Source: three-view drawing plus pictorial views. Frame: mm from the lowest corner of the part. Give positions to 0.01 mm unless a question says otherwise; leave off trailing zeros. Write each loop counter-clockwise with the first axis right and the second up, starting at its lowest first coordinate (ties: lowest second). Pieces come first, ordered by that corner, then holes.
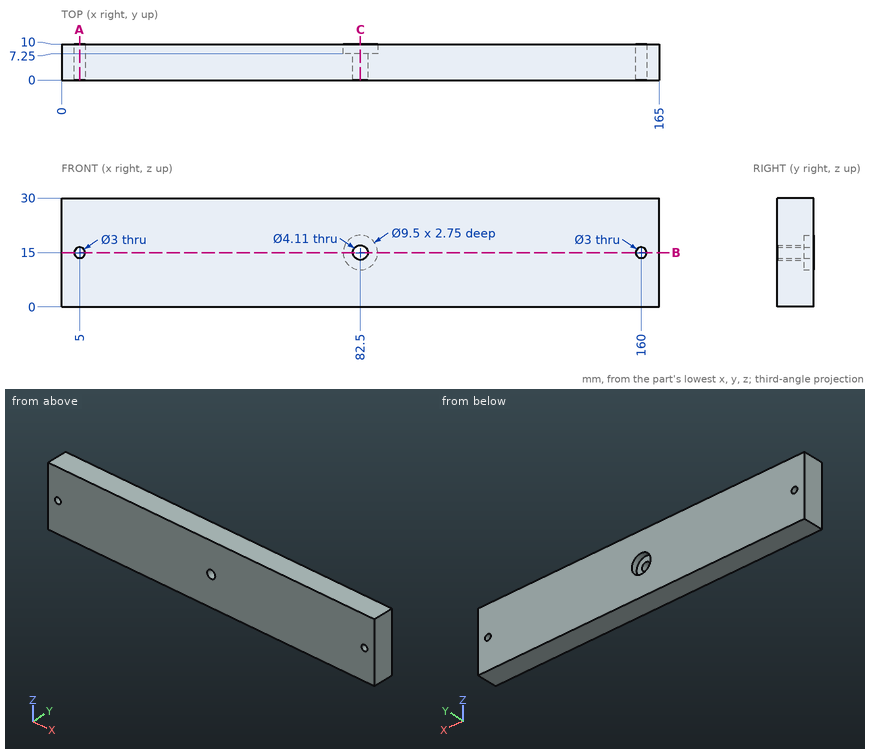
Q1. Section A-A on x = 5. Output: boundary loops of the cut face in (y, z), plus the area to 3 significant figures.
Filled sheet:
outline: (0, 0) - (10, 0) - (10, 13.5) - (0, 13.5) - close; (0, 16.5) - (10, 16.5) - (10, 30) - (0, 30) - close
area: 270 mm2
Q2. Ray query, line 1 along Z through (x, y) = (82.5, 7.85); line 2 along Z through (x, y) = (5, 6); line 3 along X through (y, z) = (9.75, 16). Return the intervals inside material, ascending.
Filled sheet:
line 1: z = 0 to 10.25, 19.75 to 30
line 2: z = 0 to 13.5, 16.5 to 30
line 3: x = 0 to 3.88, 6.12 to 77.86, 87.14 to 158.88, 161.12 to 165
Q3. Section B-B on z = 15. Output: boundary loops of the cut face in (x, y) (3 decimals).
Filled sheet:
outline: (0, 0) - (3.5, 0) - (3.5, 10) - (0, 10) - close; (6.5, 0) - (80.445, 0) - (80.445, 7.25) - (77.75, 7.25) - (77.75, 10) - (6.5, 10) - close; (84.555, 0) - (158.5, 0) - (158.5, 10) - (87.25, 10) - (87.25, 7.25) - (84.555, 7.25) - close; (161.5, 0) - (165, 0) - (165, 10) - (161.5, 10) - close
Q4. Section C-C on x = 82.5. Output: boundary loops of the cut face in (y, z) (3 decimals).
Filled sheet:
outline: (0, 0) - (10, 0) - (10, 10.25) - (7.25, 10.25) - (7.25, 12.945) - (0, 12.945) - close; (0, 17.055) - (7.25, 17.055) - (7.25, 19.75) - (10, 19.75) - (10, 30) - (0, 30) - close
Q5. Pin query (flat end, axial travel): P1, Ø7.5, axis at x = 82.5, z = 15, coming from the +Y side; P2, Ø2.5, axis at x = 160, z = 15, coming from the -Y side. Return the tip coordinate at first contact, or that it passes through.
Filled sheet:
P1: stops at y = 7.25
P2: passes through
